The listing builds one solid part. Answer for the finished solid, in the listing's coordinates (mm). Face numbers are marked on the shaded views. Round coordinates to 2 decimals unless told otherwise and drop trailing zeros. Write each loop counter-clockwise with the first axis right and the second up, starting at its lowest first coordinate (ties: lowest second). Pieces come first, ordered by that corner, then holes.
(1) A cutting plane is placed at A-A, the plane z = 5. Give the vertices of the cut face in (x, y).
(2) The mould has two halves that part along X. Classify the marked faces 1, 2, 3 and 4: +X half, -X half, draft (parallel to the pull), parting line (faces both ways), or undercut.
(3) Each of these flat-tipped pins is pushed along its axis until it touches: pin 1 Ø3 at (x, z) = (-7.5, -5) entering from +Y; pin 2 Ø1 at (x, z) = (6, -7.5) entering from -Y. Where does it stop, or does it pass through?
(4) A cutting plane is placed at C-C, the plane x = -7.5. Give the vertices of the cut face in (y, z).
(5) A cutting plane is placed at B-B, the plane y = 1.7. Give the vertices of the cut face in (x, z).
(6) Find the intervals of material crossed by probe 1 along Z at (x, y) = (-7.5, 4.6); probe 2 along X at (y, z) = (0.55, 6.25); probe 3 along X at (y, z) = (1.6, -6), in increasing order.
Autodesk Inventor part; units mm, degrees
ref_plane "YZ Plane" through (0, 0, 0) normal (1, 0, 0) x (0, 1, 0)
ref_plane "XZ Plane" through (0, 0, 0) normal (0, 1, 0) x (-1, 0, 0)
ref_plane "XY Plane" through (0, 0, 0) normal (0, 0, 1) x (1, 0, 0)
sketch "Sketch1" plane through (0, 0, 0) normal (0, 1, 0) x (-1, 0, 0)
  line L0 (-10, 14.5) -> (10, 14.5)
  line L1 (10, 14.5) -> (10, -14.5)
  line L2 (10, -14.5) -> (-10, -14.5)
  line L3 (-10, -14.5) -> (-10, 14.5)
  line L4 (-10, 14.5) -> (10, -14.5) construction
  line L5 (10, 14.5) -> (-10, -14.5) construction
  line L6 (-7.5, 5) -> (7.5, 5) construction
  line L7 (7.5, 5) -> (7.5, -5) construction
  line L8 (7.5, -5) -> (-7.5, -5) construction
  line L9 (-7.5, -5) -> (-7.5, 5) construction
  line L10 (-7.5, 5) -> (7.5, -5) construction
  line L11 (7.5, 5) -> (-7.5, -5) construction
  circle A0 centre (7.5, -5) radius 1.7
  circle A1 centre (-7.5872, -5) radius 1.7
  circle A2 centre (-7.5, 5) radius 1.7
  circle A3 centre (7.5, 5) radius 1.7
  point P0 (0, 0)
  dimension "d0" = 29
  dimension "d1" = 20
  dimension "d2" = 15
  dimension "d3" = 10
  dimension "d4" = 3.4
extrude "Extrusion1" add sketch "Sketch1" along normal blind 6
fillet "Fillet1" radius 2 4 edges at (10, 3, -14.5) (-10, 3, -14.5) (-10, 3, 14.5) (10, 3, 14.5)
properties part number "6mm XY Packer Block" material "ABS Plastic"
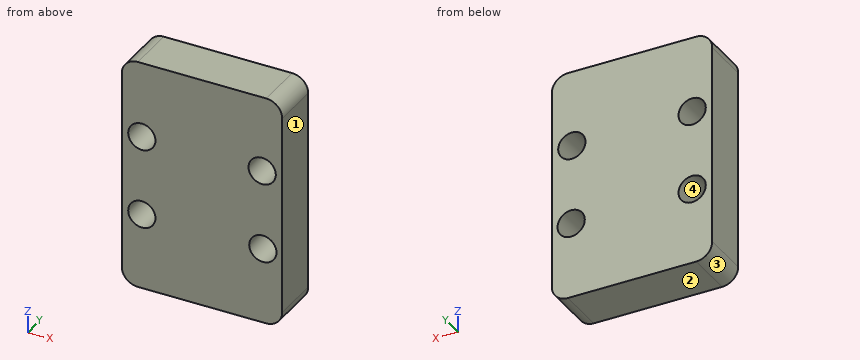
Solutions:
1. outline: (-10, 0) - (-9.2, 0) - (-9.2, 6) - (-10, 6) - close; (-5.8, 0) - (5.8, 0) - (5.8, 6) - (-5.8, 6) - close; (9.2, 0) - (10, 0) - (10, 6) - (9.2, 6) - close
2. face 1: +X half
2. face 2: draft
2. face 3: -X half
2. face 4: undercut
3. pin 1: passes through
3. pin 2: stops at y = 0
4. outline: (0, -14.5) - (6, -14.5) - (6, -6.7) - (0, -6.7) - close; (0, -3.3) - (6, -3.3) - (6, 3.3) - (0, 3.3) - close; (0, 6.7) - (6, 6.7) - (6, 14.5) - (0, 14.5) - close
5. outline: (-10, -12.5) arc R2 ccw to (-8, -14.5) - (8, -14.5) arc R2 ccw to (10, -12.5) - (10, 12.5) arc R2 ccw to (8, 14.5) - (-8, 14.5) arc R2 ccw to (-10, 12.5) - close; hole circle Ø3.4 at (-7.5, -5); hole circle Ø3.4 at (-7.5, 5); hole circle Ø3.4 at (7.5, 5); hole circle Ø3.4 at (7.59, -5)
6. probe 1: z = -14.5 to -6.7, -3.3 to 3.3, 6.7 to 14.5
6. probe 2: x = -10 to -8.65, -6.35 to 6.35, 8.65 to 10
6. probe 3: x = -10 to -8.87, -6.13 to 6.21, 8.96 to 10
